Input: part model. Units: mm. Frame: model coordinates. A direction names the side the tool comes from. Give positions to 0.01 mm unless a question says otherwise; leave off trailing zeros. Loops run counter-clockwise (first coordinate to the right, second up) from the corner with the lowest first, then second, coordinate; pieces in that order, holes last.
from build123d import *

# Parameters (mm, degrees)
F0_W     = 25.4
F0_H     = 25.4
F1_DEPTH = 6.35
F2_R     = 2.54
F3_DEPTH = 6.35
F4_R     = 2.54
F5_DEPTH = 6.35
F7_DEPTH = 5.08


with BuildPart() as f1:
    # F0 (on Right) → F1 (new body)
    with BuildSketch(Plane.YZ):
        with Locations((12.7, 12.7)):
            Rectangle(F0_W, F0_H)
    extrude(amount=F1_DEPTH)

    # F2 (on face) → F3 (cut)
    with BuildSketch(Plane.YZ.offset(6.35)):
        with Locations((12.7, 0)):
            Circle(F2_R)
        with Locations((0, 12.7)):
            Circle(F2_R)
        with Locations((12.7, 25.4)):
            Circle(F2_R)
    extrude(amount=-F3_DEPTH, mode=Mode.SUBTRACT)

    # F4 (on face) → F5 (join)
    with BuildSketch(Plane.YZ.offset(6.35)):
        with Locations((25.4, 12.7)):
            Circle(F4_R)
    extrude(amount=-F5_DEPTH)

    # F6 (on face) → F7 (cut)
    with BuildSketch(Plane.YZ.offset(6.35)):
        Polygon((21.166794, 12.697409), (17.12614, 19.701207), (9.040347, 19.703798), (4.995206, 12.702591), (9.03586, 5.698793), (17.121653, 5.696202), align=None)
    extrude(amount=-F7_DEPTH, mode=Mode.SUBTRACT)


solid = f1.part
(1) Pin query (flat end, axial travel): pin 1 Ø2 at (y, z) = (11, 14.5) entering from -X; pin 2 Ø1.5 at (x, z) = (3, 11) entering from +Y; pin 3 Ø1.9 at (x, z) = (3.5, 19) entering from +Y; pin 4 Ø2.5 at (x, y) = (4.5, 13) entering from +Z. Return the tip coordinate at first contact, or that it passes through.
Values follow:
pin 1: stops at x = 0
pin 2: stops at y = 27.76
pin 3: stops at y = 25.4
pin 4: stops at z = 23.39
(2) Reachability of faces 4 (the cylindrical face through (3.22, 12.76, 2.54)), 5 (the flat face through (3.846, 6.987, 9.25)), 6 (the flat face through (3, 25.4, 20)) from +Z, -Z, +X, -X, +Y, -Y: full face, straight path, thin tool, end or side. Return the list, or none.
Values follow:
face 4: -Z, +X, -X
face 5: +X
face 6: +Z, +X, -X, +Y
(3) Mould query, pull axis Y, two halves, no side actions, for faces 1 (the flat face through (3, 5, 25.4)), 2 (the flat face through (3.846, 19.175, 16.15)), 3 (the cylindrical face through (3.22, 2.54, 12.64)). Classes: +Y half, -Y half, draft (parallel to the pull), parting line (faces both ways), or undercut.
Values follow:
face 1: draft
face 2: undercut
face 3: -Y half
(4) Ray query, probe 1 along Y at (x, z) = (2.5, 3.25); probe 2 along Y at (x, z) = (5.5, 8); probe 3 along Z at (x, y) = (5.25, 17). Return the intervals inside material, ascending.
Values follow:
probe 1: y = 0 to 25.4
probe 2: y = 0 to 7.71, 18.45 to 25.4
probe 3: z = 0 to 5.7, 19.7 to 25.4
(5) Cut plane D-D (y = 14.5). Return the cut outline in (x, z), and give its area (3 significant figures).
Values follow:
outline: (0, 1.79) - (6.35, 1.79) - (6.35, 5.7) - (1.27, 5.7) - (1.27, 19.7) - (6.35, 19.7) - (6.35, 23.61) - (0, 23.61) - close
area: 67.4 mm2
(6) Cut plane A-A (x = 2). Return the cut outline in (y, z).
Values follow:
outline: (0, 0) - (10.16, 0) arc R2.54 cw to (15.24, 0) - (25.4, 0) - (25.4, 10.16) arc R2.54 ccw to (25.4, 15.24) - (25.4, 25.4) - (15.24, 25.4) arc R2.54 cw to (10.16, 25.4) - (0, 25.4) - (0, 15.24) arc R2.54 cw to (0, 10.16) - close; hole (5, 12.7) - (9.04, 5.7) - (17.12, 5.7) - (21.17, 12.7) - (17.13, 19.7) - (9.04, 19.7) - close
(7) Cut plane B-B (z = 1.75). Return the cut outline in (x, y).
Values follow:
outline: (0, 0) - (6.35, 0) - (6.35, 10.86) - (0, 10.86) - close; (0, 14.54) - (6.35, 14.54) - (6.35, 25.4) - (0, 25.4) - close
(8) Cut plane C-C (y = 2). Return the cut outline in (x, z).
Values follow:
outline: (0, 0) - (6.35, 0) - (6.35, 11.13) - (0, 11.13) - close; (0, 14.27) - (6.35, 14.27) - (6.35, 25.4) - (0, 25.4) - close
